Could you check a few things on this model? Use its own coordinates, in mm. Round coordinates to 2 decimals unless told otherwise and drop trailing zeros. Write each loop counter-clockwise with the first axis right and the second up, starting at its lowest first coordinate (ties: lowest second). Pieces come first, ordered by that corner, then holes.
```python
from build123d import *

# Parameters (mm, degrees)
SKETCH_1_W      = 2100
SKETCH_1_H      = 210
EXTRUDE_1_DEPTH = 5.4
SKETCH_2_W      = 75
SKETCH_2_H      = 30
SKETCH_2_W_2    = 85
EXTRUDE_2_DEPTH = 18
SKETCH_4_W      = 1968
SKETCH_4_H      = 182
EXTRUDE_3_DEPTH = 0.2


with BuildPart() as part:
    # 草图1 → 凸台-拉伸1 (new body)
    with BuildSketch(Plane.XY):
        with Locations((1050, 105)):
            Rectangle(SKETCH_1_W, SKETCH_1_H)
    extrude(amount=EXTRUDE_1_DEPTH)

    # 草图2 → 凸台-拉伸2 (add)
    with BuildSketch(Plane.XY.offset(5.4)):
        with Locations((277.5, 15)):
            Rectangle(SKETCH_2_W, SKETCH_2_H)
        with Locations((677.5, 15)):
            Rectangle(SKETCH_2_W_2, SKETCH_2_H)
    extrude(amount=EXTRUDE_2_DEPTH)

    # 草图4 → 凸台-拉伸3 (add)
    with BuildSketch(Plane(origin=(0, 0, 0), x_dir=(-1, 0, 0), z_dir=(0, 0, -1))):
        with Locations((-1050, 109)):
            Rectangle(SKETCH_4_W, SKETCH_4_H)
    extrude(amount=EXTRUDE_3_DEPTH)


solid = part.part
```
Q1. If I drill on L1, parallel to Z at x = 1960, y = 48; L2, parallel to Y at x = 698, z = 16.75; L3, parallel to Z at x = 772, y = 11, over which ranges is the centre line in solid material (lowest first)?
Q2. I'm going to push flat-ended pins straight in: pin 1 Ø1 at (y, z) = (82.5, 7) entering from +X; pin 2 Ø3 at (x, y) = (449, 27.5) entering from +Z; pin 3 Ø9 at (x, z) = (667, 16.5) entering from +Y. Where does each tip first touch, or does it pass through?
Q3. Imagine slicing it at C-C, the plane x = 987. Write out the boundary of the cut face in (y, z), then the cut area to 3 significant figures.
Q4. Imagine slicing it at B-B, the plane y = 162. Write out the boundary of the cut face in (x, z).
Q5. Imagine slicing it at A-A, the plane z = 19. Write out the boundary of the cut face in (x, y), then the cut area to 3 significant figures.
Results found:
1. L1: z = -0.2 to 5.4
1. L2: y = 0 to 30
1. L3: z = 0 to 5.4
2. pin 1: passes through
2. pin 2: stops at z = 5.4
2. pin 3: stops at y = 30
3. outline: (0, 0) - (18, 0) - (18, -0.2) - (200, -0.2) - (200, 0) - (210, 0) - (210, 5.4) - (0, 5.4) - close
3. area: 1,170 mm2
4. outline: (0, 0) - (66, 0) - (66, -0.2) - (2034, -0.2) - (2034, 0) - (2100, 0) - (2100, 5.4) - (0, 5.4) - close
5. outline: (240, 0) - (315, 0) - (315, 30) - (240, 30) - close; (635, 0) - (720, 0) - (720, 30) - (635, 30) - close
5. area: 4,800 mm2
